from build123d import *

# Parameters (mm, degrees)
SKETCH4_R           = 5.5
SKETCH4_R_2         = 1.5
BOSS_EXTRUDE2_DEPTH = 4
CUT_EXTRUDE1_START  = -2
CUT_EXTRUDE1_DEPTH  = 2


with BuildPart() as part:
    # Sketch4 → Boss-Extrude2 (new body)
    with BuildSketch(Plane.XY):
        with BuildLine():
            Line((28, 3.1), (26, 3.1))
            ThreePointArc((26, 3.1), (25.707834138, 3.086201405), (25.418269231, 3.044928458))
            ThreePointArc((25.418269231, 3.044928458), (18.101933598, 18.101933598), (3.044928458, 25.418269231))
            ThreePointArc((3.044928458, 25.418269231), (3.086201405, 25.707834138), (3.1, 26))
            Line((3.1, 26), (3.1, 28))
            ThreePointArc((3.1, 28), (0, 31.1), (-3.1, 28))
            Line((-3.1, 28), (-3.1, 26))
            ThreePointArc((-3.1, 26), (-3.086201405, 25.707834138), (-3.044928458, 25.418269231))
            ThreePointArc((-3.044928458, 25.418269231), (-18.101933598, 18.101933598), (-25.418269231, 3.044928458))
            ThreePointArc((-25.418269231, 3.044928458), (-25.707834138, 3.086201405), (-26, 3.1))
            Line((-26, 3.1), (-28, 3.1))
            ThreePointArc((-28, 3.1), (-31.1, 0), (-28, -3.1))
            Line((-28, -3.1), (-26, -3.1))
            ThreePointArc((-26, -3.1), (-25.707834138, -3.086201405), (-25.418269231, -3.044928458))
            ThreePointArc((-25.418269231, -3.044928458), (-18.101933598, -18.101933598), (-3.044928458, -25.418269231))
            ThreePointArc((-3.044928458, -25.418269231), (-3.086201405, -25.707834138), (-3.1, -26))
            Line((-3.1, -26), (-3.1, -28))
            ThreePointArc((-3.1, -28), (0, -31.1), (3.1, -28))
            Line((3.1, -28), (3.1, -26))
            ThreePointArc((3.1, -26), (3.086201405, -25.707834138), (3.044928458, -25.418269231))
            ThreePointArc((3.044928458, -25.418269231), (18.101933598, -18.101933598), (25.418269231, -3.044928458))
            ThreePointArc((25.418269231, -3.044928458), (25.707834138, -3.086201405), (26, -3.1))
            Line((26, -3.1), (28, -3.1))
            ThreePointArc((28, -3.1), (31.1, 0), (28, 3.1))
        make_face()
        Circle(SKETCH4_R, mode=Mode.SUBTRACT)
        with Locations((-28, 0)):
            Circle(SKETCH4_R_2, mode=Mode.SUBTRACT)
        with Locations((0, 28)):
            Circle(SKETCH4_R_2, mode=Mode.SUBTRACT)
        with Locations((28, 0)):
            Circle(SKETCH4_R_2, mode=Mode.SUBTRACT)
        with Locations((0, -28)):
            Circle(SKETCH4_R_2, mode=Mode.SUBTRACT)
    extrude(amount=BOSS_EXTRUDE2_DEPTH)

    # Sketch5 → Cut-Extrude1 (cut)
    with BuildSketch(Plane.XY.offset(4).offset(CUT_EXTRUDE1_START)):
        with BuildLine():
            Line((-25.418269231, -3.044928458), (-2.892398424, 4.678037126))
            Line((-2.892398424, 4.678037126), (9.11402937, 23.92267687))
            ThreePointArc((9.11402937, 23.92267687), (13.159458029, 21.958794693), (16.798827647, 19.317333918))
            Line((16.798827647, 19.317333918), (5.5, 0))
            Line((5.5, 0), (17.104166933, -19.047505704))
            ThreePointArc((17.104166933, -19.047505704), (13.991450126, -21.438267733), (10.549853348, -23.325106524))
            Line((10.549853348, -23.325106524), (0, -5.5))
            Line((0, -5.5), (-22.195690438, -12.755834977))
            ThreePointArc((-22.195690438, -12.755834977), (-24.297072153, -8.063019583), (-25.418269231, -3.044928458))
        make_face()
    extrude(amount=CUT_EXTRUDE1_DEPTH, mode=Mode.SUBTRACT)


solid = part.part
Design review of the part built by this model. Coordinates are the model's own, in mm. A direction names the side the tool comes from. Coordinates: 2 decimals unless noted, no trailing zeros. Order: outer loops, then holes, each group sorted by start corner. A loop starts at its lowest first (then second) coordinate and runs counter-clockwise, first axis right, second up. Notation, with made-up numbers: (77.25, 71) -> (105.25, 71) arc R12 ccw to (105.25, 82) -> close; hole circle Ø2 at (-1, 46.5). An arc over 180 degrees is marked (long way). Use one line per item in the form item = value. Start each with the question number.
(1) Insertion check: pin 1 (1.6 mm diameter, centred on y = 27, z = 2.5, fed in from -X); pin 2 (2 mm diameter, centred on y = -27.5, z = 2, fed in from +X); pin 3 (2 mm diameter, centred on x = 27, z = 1.5, fed in from -Y); pin 4 (2.5 mm diameter, centred on x = 0, y = 28, fed in from -Z). Each pin has a flat end and moves straight along its axis. Give the tip position at first contact, or say it passes through.
(2) For probe 1 along Y at (x, z) = (0, 1.3); probe 2 along Y at (x, z) = (0, 2.55); probe 3 along Y at (x, z) = (-2, 1.6), list the stretches that pass through material, from the lowest coordinate up.
(3) Add section B-B on x = -17.5. State the section outline as (y, z) points, plus the area to 3 significant figures.
(4) For faces 1 (the flat face through (-3.1, 27, 2)), 2 (the flat face through (-3.1, -27, 2)), 3 (the flat face through (9, -11, 2)), list the 3-axis set-ups (+Z, -Z, +X, -X, +Y, -Y) from which the entire face can be reached by the end or side of a thin tool; tool diameter is ignored.
(5) The part is to be moulded in two halves that separate along Y. For faces 4 (the cylindrical face through (0.1, 31.1, 2)), 5 (the flat face through (11.22, -9.39, 2.99)), 6 (the cylindrical face through (-0.195, -26.513, 1.972)), 7 (the flat face through (-6, -18, 4)), say which applies: +Y half, -Y half, draft (parallel to the pull), parting line (faces both ways), or undercut.
(6) Add section A-A on z = 0.85. Give the number of separate pieces and of enclosed holes in the cut face, plus the area to 3 significant figures.
Answer block:
q1.pin_1 = -3.1
q1.pin_2 = 3.1
q1.pin_3 = -3.1
q1.pin_4 = through
q2.probe_1 = -31.1 to -29.5, -26.5 to -5.5, 5.5 to 26.5, 29.5 to 31.1
q2.probe_2 = -31.1 to -29.5, -26.5 to -5.5, 9.31 to 26.5, 29.5 to 31.1
q2.probe_3 = -30.37 to -5.12, 5.12 to 30.37
q3.outline = (-18.68, 0) -> (18.68, 0) -> (18.68, 4) -> (-0.33, 4) -> (-0.33, 2) -> (-11.22, 2) -> (-11.22, 4) -> (-18.68, 4) -> close
q3.area = 128 mm²
q4.face_1 = +Z, -Z, -X, +Y
q4.face_2 = +Z, -Z, -X, -Y
q4.face_3 = +Z
q5.face_4 = +Y half
q5.face_5 = undercut
q5.face_6 = undercut
q5.face_7 = draft
q6.separate_pieces = 1
q6.enclosed_holes = 5
q6.area = 2,060 mm²
